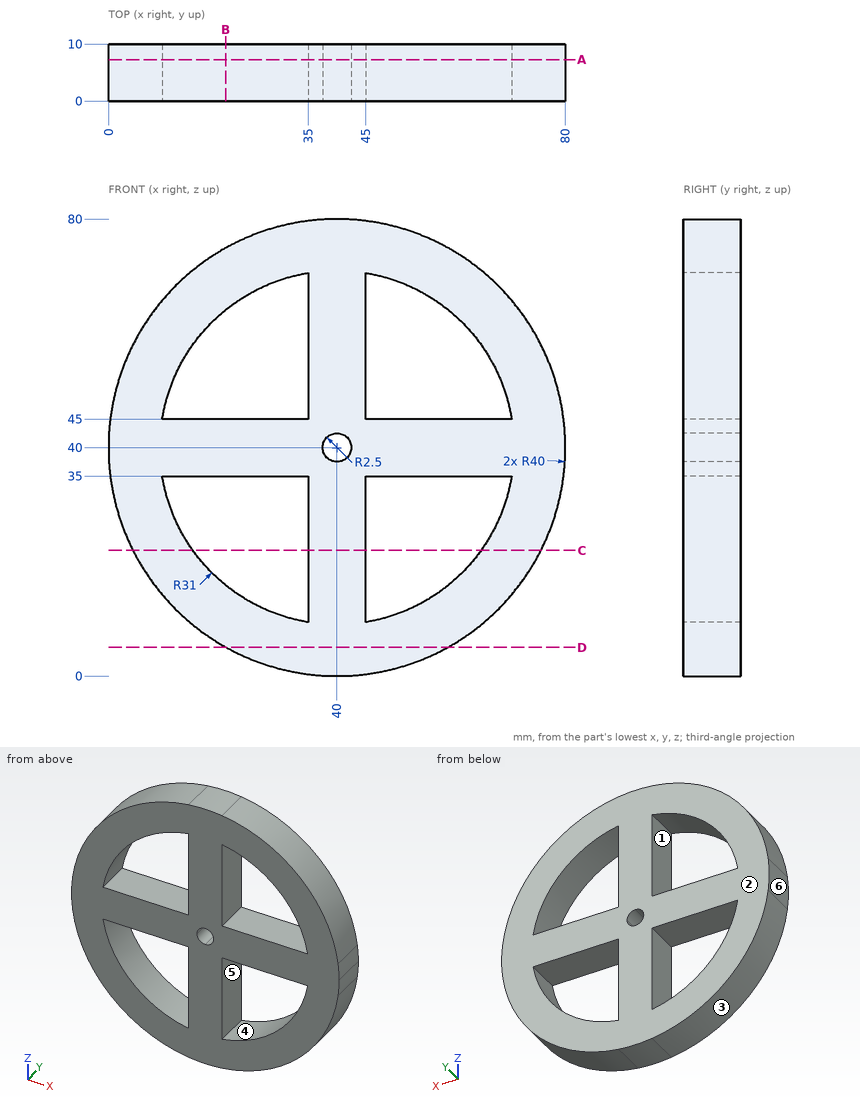
Input: dimensioned drawing with shaded views. Units: mm. Origin: part minimum x, y, z. A direction names the side the tool comes from. Coordinates: 2 decimals unless noted, no trailing zeros. Order: outer loops, then holes, each group sorted by start corner. A loop starts at its lowest first (then second) coordinate and runs counter-clockwise, first axis right, second up.
1. Cut plane B-B, the plane x = 20.5. Return loops of the section in (y, z) (1 decimal).
Checked values:
outline: (0, 5.1) - (10, 5.1) - (10, 15.9) - (0, 15.9) - close; (0, 35) - (10, 35) - (10, 45) - (0, 45) - close; (0, 64.1) - (10, 64.1) - (10, 74.9) - (0, 74.9) - close
2. Contact query for flat-ended pins moving along their axis: P1, Ø6, axis at y = 8.5, z = 64, coming from the -X side; P2, Ø3, axis at x = 54, y = 6, coming from the +Z side; P3, Ø3, axis at x = 23, y = 2.5, coming from the -Z side (1 decimal). Output: stop coordinate, or through.
Checked values:
P1: stops at x = 5.96
P2: stops at z = 78
P3: stops at z = 3.1
3. Cut plane A-A, the plane y = 7.25. Return loops of the section in (x, z).
Checked values:
outline: (0.31, 35) arc R40 ccw to (35, 0.31) arc R40 ccw to (45, 0.31) arc R40 ccw to (79.69, 35) arc R40 ccw to (80, 40) arc R40 ccw to (79.69, 45) arc R40 ccw to (45, 79.69) arc R40 ccw to (35, 79.69) arc R40 ccw to (0.31, 45) arc R40 ccw to start; hole (9.41, 35) arc R31 ccw to (35, 9.41) - (35, 35) - close; hole (9.41, 45) - (35, 45) - (35, 70.59) arc R31 ccw to start; hole circle Ø5 at (40, 40); hole (45, 9.41) arc R31 ccw to (70.59, 35) - (45, 35) - close; hole (45, 45) - (70.59, 45) arc R31 ccw to (45, 70.59) - close
4. Cut plane D-D, the plane z = 5. Return loops of the section in (x, y) (1 decimal), plus the area to 3 significant figures.
Checked values:
outline: (20.6, 0) - (59.4, 0) - (59.4, 10) - (20.6, 10) - close
area: 387 mm2
5. Cut plane C-C, the plane z = 22. Return loops of the section in (x, y), plus the area to 3 significant figures.
Checked values:
outline: (4.28, 0) - (14.76, 0) - (14.76, 10) - (4.28, 10) - close; (35, 0) - (45, 0) - (45, 10) - (35, 10) - close; (65.24, 0) - (75.72, 0) - (75.72, 10) - (65.24, 10) - close
area: 310 mm2
6. Access query for the marked faces 5 and 6. Directions: +Z, -Z, +X, -X, +Y, -Y. A direction counts if a zero-diameter tool reaches every point of the face in a straight line with its end or side. Return the directions, or none.
Checked values:
face 5: +Y, -Y
face 6: -X, +Y, -Y
7. Ray query, line 1 along X through (y, z) = (2.5, 30.5) (1 decimal); line 2 along X through (y, z) = (8, 23.5) (1 decimal); line 3 along Z through (x, y) = (48, 4.25). Return the intervals inside material, ascending.
Checked values:
line 1: x = 1.1 to 10.5, 35 to 45, 69.5 to 78.9
line 2: x = 3.6 to 13.8, 35 to 45, 66.2 to 76.4
line 3: z = 0.81 to 10.05, 35 to 45, 69.95 to 79.19
8. Draft query along Z for the marked faces 1, 2, 3 and 4. Return one class per face: +Z half, -Z half, draft (parallel to the pull), parting line (faces both ways), or undercut.
Checked values:
face 1: undercut
face 2: draft
face 3: -Z half
face 4: undercut
